Answer from the drawing. Dimensions are ordinates in mm from the lowest x, y and z of the part. A direction names the side the tool comes from. Give positions to 0.01 mm unless a question says otherwise; leave off trailing zeros. Order: outer loops, then holes, each group sorted by start corner. A loop starts at its lowest first (then second) coordinate and runs counter-clockwise, first axis right, second up.
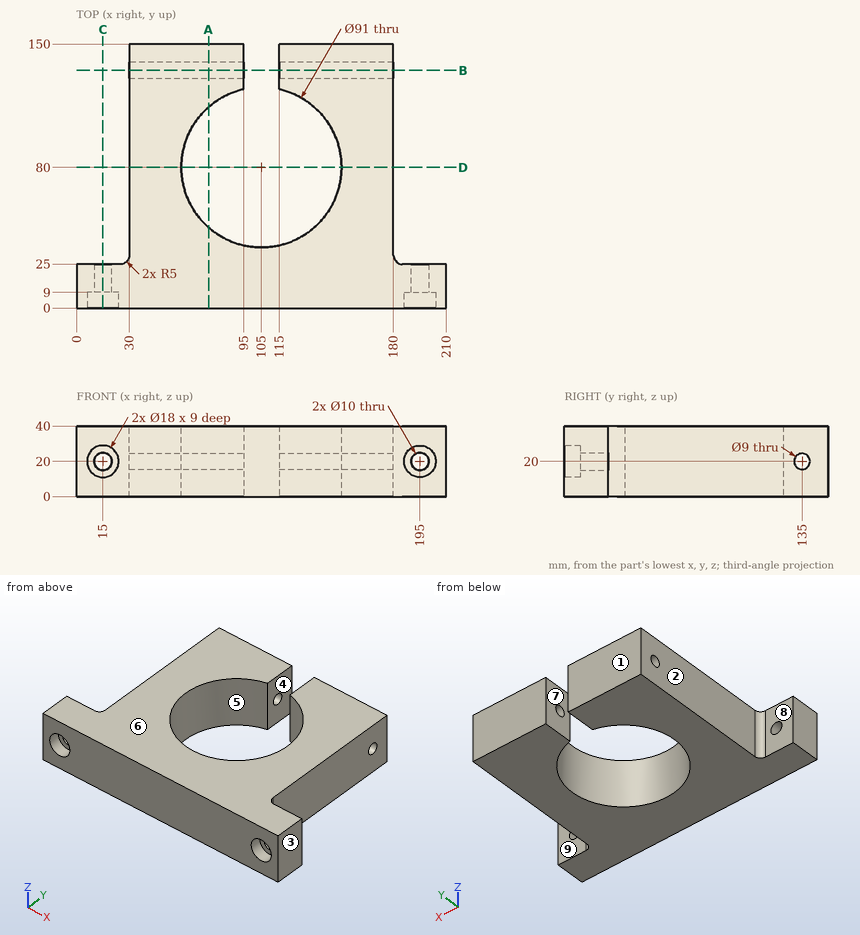
1) The part is cut by section B-B on y = 135. Determine the outline of the cut face in (x, z).
Final values:
outline: (30, 0) - (95, 0) - (95, 15.5) - (30, 15.5) - close; (30, 24.5) - (95, 24.5) - (95, 40) - (30, 40) - close; (115, 0) - (180, 0) - (180, 15.5) - (115, 15.5) - close; (115, 24.5) - (180, 24.5) - (180, 40) - (115, 40) - close
2) The part is cut by section A-A on x = 75. Determine the outline of the cut face in (y, z).
Final values:
outline: (0, 0) - (45.79, 0) - (45.79, 40) - (0, 40) - close; (114.21, 0) - (150, 0) - (150, 40) - (114.21, 40) - close; hole circle Ø9 at (135, 20)
3) Consider L1, parallel to X at y = 19, z = 20; L2, parallel to Z at x = 15, y = 2.75; L3, parallel to Z at x = 15, y = 14. Determine where each line is inside the solid, lowest interval first.
Final values:
L1: x = 0 to 10, 20 to 190, 200 to 210
L2: z = 0 to 11, 29 to 40
L3: z = 0 to 15, 25 to 40
4) A tool of negligible diameter and unlimited length cuts with its end or side. For the marked faces 5, 6, 7, 8 and 9, from which of +Z, -Z, +X, -X, +Y, -Y can it reach the whole face along a straight path? Write none if from no direction.
Final values:
face 5: +Z, -Z
face 6: +Z, +X, -X, +Y, -Y
face 7: +Z, -Z, +Y
face 8: +Z, -Z, -X, +Y
face 9: +Z, -Z, +X, +Y
5) Given pin 1 (8 mm diameter, centred on x = 134, y = 111, fed in from -Z); pin 2 (13 mm diameter, centred on y = 135.5, z = 29, fed in from -X); pin 3 (4 mm diameter, centred on y = 109, z = 7.5, fed in from +X); pin 4 (12.5 mm diameter, centred on x = 191.5, z = 13, fed in from +Y), each flat-ended and moving along its own axis, determine where each tip first touches the part or whether it passes through.
Final values:
pin 1: stops at z = 0
pin 2: stops at x = 30
pin 3: stops at x = 180
pin 4: stops at y = 25
6) For a pull along X with two mould halves and no side action, classify the marked faces 1, 2, 3 and 4 as released by +X, released by -X, zero draft, split by the parting line, or undercut.
Final values:
face 1: zero draft
face 2: released by -X
face 3: released by +X
face 4: undercut
7) The part is cut by section C-C on x = 15. Determine the outline of the cut face in (y, z).
Final values:
outline: (0, 0) - (25, 0) - (25, 15) - (9, 15) - (9, 11) - (0, 11) - close; (0, 29) - (9, 29) - (9, 25) - (25, 25) - (25, 40) - (0, 40) - close
8) The part is cut by section D-D on y = 80. Determine the outline of the cut face in (x, z), and give its area (3 significant figures).
Final values:
outline: (30, 0) - (59.5, 0) - (59.5, 40) - (30, 40) - close; (150.5, 0) - (180, 0) - (180, 40) - (150.5, 40) - close
area: 2,360 mm2
